```python
from build123d import *

# Parameters (mm, degrees)
F0_W      = 250
F0_H      = 10.25
F0_H_2    = 35
F0_R      = 1.5
F0_W_2    = 18
F0_H_3    = 5.08
F1_DEPTH  = 5.8
F1_FACE_W = 50
F1_FACE_H = 5.8
F2_DEPTH  = 25


with BuildPart() as f1:
    # F0 (on Front) → F1 (new body)
    with BuildSketch(Plane.XZ):
        with Locations((2.281713, 50.611829)):
            Rectangle(F0_W, F0_H)
        with Locations((2.281713, 27.986829)):
            Rectangle(F0_W, F0_H_2)
        with Locations((-109.911287, 39.236829)):
            Circle(F0_R, mode=Mode.SUBTRACT)
        with BuildLine():
            Line((127.281713, 0.236829), (127.281713, 10.486829))
            Line((127.281713, 10.486829), (-122.718287, 10.486829))
            Line((-122.718287, 10.486829), (-122.718287, 0.236829))
            Line((-122.718287, 0.236829), (-111.029321, 0.236829))
            ThreePointArc((-111.029321, 0.236829), (-110.44652, 2.638087), (-108.411287, 1.236829))
            ThreePointArc((-108.411287, 1.236829), (-108.510028, 0.701596), (-108.793253, 0.236829))
            Line((-108.793253, 0.236829), (78.874297, 0.236829))
            Line((78.874297, 0.236829), (78.874297, 5.228526))
            Line((78.874297, 5.228526), (96.874297, 5.228526))
            Line((96.874297, 5.228526), (96.874297, 0.236829))
            Line((96.874297, 0.236829), (127.281713, 0.236829))
        make_face()
        with BuildLine():
            Line((127.281713, -59.514336), (127.281713, 0.236829))
            Line((127.281713, 0.236829), (96.874297, 0.236829))
            Line((96.874297, 0.236829), (96.874297, 0.148526))
            Line((96.874297, 0.148526), (78.874297, 0.148526))
            Line((78.874297, 0.148526), (78.874297, 0.236829))
            Line((78.874297, 0.236829), (-108.793253, 0.236829))
            ThreePointArc((-108.793253, 0.236829), (-109.911287, -0.263171), (-111.029321, 0.236829))
            Line((-111.029321, 0.236829), (-122.718287, 0.236829))
            Line((-122.718287, 0.236829), (-122.718287, -19.263171))
            ThreePointArc((-122.718287, -19.263171), (-101.334346, -13.710596), (-79.665576, -9.401492))
            ThreePointArc((-79.665576, -9.401492), (-8.261862, -4.127499), (62.874297, -12.248605))
            Line((62.874297, -12.248605), (62.874297, -65.755888))
            Line((62.874297, -65.755888), (62.874297, -92.638836))
            Line((62.874297, -92.638836), (62.874297, -119.263171))
            Line((62.874297, -119.263171), (112.874297, -119.263171))
            Line((112.874297, -119.263171), (127.281713, -59.514336))
        make_face()
        with Locations((87.874297, -97.311474)):
            Rectangle(F0_W_2, F0_H_3, mode=Mode.SUBTRACT)
        with Locations((87.874297, -47.311474)):
            Rectangle(F0_W_2, F0_H_3, mode=Mode.SUBTRACT)
        with BuildLine():
            ThreePointArc((-79.665576, -9.401492), (-101.334346, -13.710596), (-122.718287, -19.263171))
            Line((-122.718287, -19.263171), (62.874297, -92.638836))
            Line((62.874297, -92.638836), (62.874297, -65.755888))
            Line((62.874297, -65.755888), (-79.665576, -9.401492))
        make_face()
    extrude(amount=F1_DEPTH)

    # F1_face (on face) → F2 (join)
    with BuildSketch(Plane(origin=(87.874297, -2.9, -119.263171), x_dir=(1, 0, 0), z_dir=(0, 0, -1))):
        Rectangle(F1_FACE_W, F1_FACE_H)
    extrude(amount=F2_DEPTH)


solid = f1.part
```
Source: CAD feature listing. Evaluate the final solid. Frame: model axes, mm. A direction names the side the tool comes from. Round coordinates to 2 decimals unless told otherwise and drop trailing zeros. Write each loop counter-clockwise with the first axis right and the second up, starting at its lowest first coordinate (ties: lowest second). Pieces come first, ordered by that corner, then holes. Notation, with made-up numbers: M 39.25,2 L 92.25,2 A33 ccw 92.25,32 Z; hole C -9.5,-1.5 d1. An arc over 180 degrees is marked long. Answer as a JSON object with one key per item and string values. Group by question number.
(1) First-contact query: pin 1 (2.5 mm diameter, centred on x = -109.91, z = 39.24, fed in from +Y); pin 2 (1.7 mm diameter, centred on y = -2, z = -130, fed in from +X); pin 3 (3 mm diameter, centred on x = -63.5, y = -4.5, fed in from -Z); pin 4 (10 mm diameter, centred on x = 99, z = -0.5, fed in from +Y). Flat tips, straight axial feed; report the tip coordinate or a pass-through.
(2) Reachability of faces 1 (the flat face through (62.874, -3, -118)), 2 (the flat face through (112.874, -3, -132)), 3 (the flat face through (96.874, -3, -97)) from +Z, -Z, +X, -X, +Y, -Y: full face, straight path, thin tool, end or side. Return the list, or none.
(3) Section query C-C on y = -1. Output: boundary loops of the cut face in (x, z), then the cut area to 3 significant figures.
(4) Section query D-D on z = -35. Output: boundary loops of the cut face in (x, y).
(5) Ray query, line 1 (Z direction, x = 83, y = -3.35); line 2 (X direction, y = -2.3, z = -127.5); line 3 (Z direction, x = -109.5, y = -4.35). Return the intervals inside material, ascending. Write a range as [from, to].
(6) Mould query, pull axis X, two halves, no side actions, for faces 4 (the flat face through (88, -3, 5.229)), 5 (the flat face through (-122.718, -3, 19)), 6 (the flat face through (28, 0, 2)). Classes: +X half, -X half, draft (parallel to the pull), parting line (faces both ways), or undercut.
(7) Section query A-A on x = -0.5. Output: boundary loops of the cut face in (y, z), then the cut area to 3 significant figures.
(8) Section query B-B on x = 91. Output: boundary loops of the cut face in (y, z).
Computed values:
{
 "1": {"pin 1": "through", "pin 2": "x = 112.87", "pin 3": "z = -43.27", "pin 4": "y = 0"},
 "2": {"face 1": "-Z, -X, +Y, -Y", "face 2": "-Z, +X, +Y, -Y", "face 3": "+Y, -Y"},
 "3": {"outline": "M -122.72,-19.26 L 62.87,-92.64 L 62.87,-144.26 L 112.87,-144.26 L 112.87,-119.26 L 127.28,-59.51 L 127.28,55.74 L -122.72,55.74 Z; hole C -109.91,39.24 d3; hole M -108.79,0.24 A1.5 ccw -108.41,1.24 A1.5 ccw long Z; hole M -79.67,-9.4 L 62.87,-65.76 L 62.87,-12.25 A382.62 ccw Z; hole M 78.87,-99.85 L 96.87,-99.85 L 96.87,-94.77 L 78.87,-94.77 Z; hole M 78.87,-49.85 L 96.87,-49.85 L 96.87,-44.77 L 78.87,-44.77 Z; hole M 78.87,0.15 L 96.87,0.15 L 96.87,5.23 L 78.87,5.23 Z", "area": "28,100 mm^2"},
 "4": {"outline": "M -82.91,-5.8 L -14.92,-5.8 L -14.92,0 L -82.91,0 Z; M 62.87,-5.8 L 127.28,-5.8 L 127.28,0 L 62.87,0 Z"},
 "5": {"line 1": "[-144.26, -99.85], [-94.77, -49.85], [-44.77, 0.15], [5.23, 55.74]", "line 2": "[62.87, 112.87]", "line 3": "[-24.49, -0.21], [2.68, 37.79], [40.68, 55.74]"},
 "6": {"face 4": "undercut", "face 5": "-X half", "face 6": "draft"},
 "7": {"outline": "M -5.8,-67.58 L 0,-67.58 L 0,-40.7 L -5.8,-40.7 Z; M -5.8,-4.36 L 0,-4.36 L 0,55.74 L -5.8,55.74 Z", "area": "504 mm^2"},
 "8": {"outline": "M -5.8,-144.26 L 0,-144.26 L 0,-99.85 L -5.8,-99.85 Z; M -5.8,-94.77 L 0,-94.77 L 0,-49.85 L -5.8,-49.85 Z; M -5.8,-44.77 L 0,-44.77 L 0,0.15 L -5.8,0.15 Z; M -5.8,5.23 L 0,5.23 L 0,55.74 L -5.8,55.74 Z"}
}
